Check sheet for the modelled part. Datum: model origin and axes. Units: mm. Face numbers are marked on the shaded views. A direction names the side the tool comes from. Coordinates: 2 decimals unless noted, no trailing zeros. Loops run counter-clockwise (first coordinate to the right, second up) from the corner with the lowest first, then second, coordinate; pieces in that order, holes last. Notation, with made-up numbers: M -38,70 L -6,70 A14 cw -6,92 Z; hole C 32,63 d10. An arc over 180 degrees is marked long. Write each question's results on one line, items separated by ' | '. Start each with the question number.
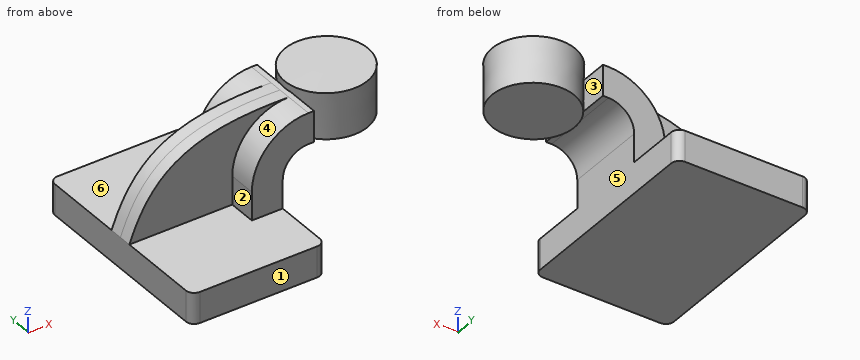
from build123d import *

# Parameters (mm, degrees)
F1_DEPTH = 63.5
F2_DEPTH = 25.4
F3_DEPTH = 7.9375
F5_R     = 5.08


with BuildPart() as f1:
    # F0 (on Front) → F1 (new body, symmetric)
    with BuildSketch(Plane.XZ):
        Polygon((22.2249999642, 9.525), (-41.275, 9.525), (-41.275, -9.525), (41.275, -9.525), (41.275, 9.525), align=None)
    extrude(amount=F1_DEPTH, both=True)

    # F0 (on Front) → F2 (join, symmetric)
    with BuildSketch(Plane.XZ):
        with BuildLine():
            Line((22.2249999642, 27.0002), (22.2249999642, 9.525))
            Line((22.2249999642, 9.525), (41.275, 9.525))
            Line((41.275, 9.525), (41.275, 27.0002))
            ThreePointArc((41.275, 27.0002), (45.9246798487, 38.2255201513), (57.15, 42.8752))
            Line((57.15, 42.8752), (60.587947001, 42.8752))
            Line((60.587947001, 42.8752), (60.587947001, 61.9252000358))
            Line((60.587947001, 61.9252000358), (57.15, 61.9252000358))
            ThreePointArc((57.15, 61.9252000358), (32.4542956418, 51.6959043582), (22.2249999642, 27.0002))
        make_face()
    extrude(amount=F2_DEPTH, both=True)

    # F0 (on Front) → F3 (join, symmetric)
    with BuildSketch(Plane.XZ):
        with BuildLine():
            add(Edge.make_bspline(
                [(-41.275, 9.525), (-27.342395857, 48.1158420444), (-3.4818400163, 63.5879263282), (57.15, 61.9252000358)],
                knots=[0, 0, 0, 0, 111.5045361803, 111.5045361803, 111.5045361803, 111.5045361803], degree=3))
            Line((-41.275, 9.525), (22.2249999642, 9.525))
            Line((22.2249999642, 9.525), (22.2249999642, 27.0002))
            ThreePointArc((22.2249999642, 27.0002), (32.4542956418, 51.6959043582), (57.15, 61.9252000358))
        make_face()
    extrude(amount=F3_DEPTH, both=True)

    # F0 (on Front) → F4 (revolve)
    with BuildSketch(Plane.XZ):
        Polygon((111.387947001, 66.675), (85.725, 66.675), (85.987947001, 38.1), (111.387947001, 38.1), align=None)
    revolve(axis=Axis((85.8564735005, 0, 52.3875), (-0.0092016052, 0, 0.9999576643)))

    # F5
    f5_edges = [f1.edges().sort_by_distance(p)[0] for p in [
        (41.275, -63.5, 0),
        (-41.275, -63.5, 0),
        (41.275, 63.5, 0),
        (-41.275, 63.5, 0),
    ]]
    fillet(f5_edges, radius=F5_R)


solid = f1.part
Item 1: Tool access check on the marked faces 4, 5 and 6. Record the directions out of +Z, -Z, +X, -X, +Y, -Y that give a thin tool (end or side, any length) a straight path to the whole face; none if there is none.
Item 2: Section check B-B (y = -42). Record the cut outline in (x, z) (3 decimals), plus the area to 3 significant figures.
Item 3: Section check A-A (z = 3). Record the cut outline in (x, y) (3 decimals), plus the area to 3 significant figures.
Item 4: Depth check by flat-ended pin: P1, Ø9.5, axis at y = -19.5, z = 54.5, coming from the +X side; P2, Ø4, axis at x = 59.5, y = -4.5, coming from the +Z side; P3, Ø11.5, axis at x = 49, z = 38.5, coming from the -Y side. Enter the tip coordinate at first touch or a pass-through.
Item 5: Thickness scan on line 1 (X direction, y = 27, z = -4.5) (3 decimals); line 2 (Y direction, x = 5.5, z = 11); line 3 (X direction, y = 13, z = 15) (3 decimals). Record the ranges inside material, lowest first.
Item 6: Release check for a two-part mould opening along X. For the marked faces 1, 2 and 3 record: +X half, -X half, draft (parallel to the pull), parting line (faces both ways), or undercut.
Computed values:
1) face 4: +Z, -X, -Y | face 5: -Z, +X, +Y, -Y | face 6: +Z, -X, +Y
2) outline: M -41.275,-9.525 L 41.275,-9.525 L 41.275,9.525 L -41.275,9.525 Z | area: 1,570 mm²
3) outline: M -41.275,-58.42 A5.08 ccw -36.195,-63.5 L 36.195,-63.5 A5.08 ccw 41.275,-58.42 L 41.275,58.42 A5.08 ccw 36.195,63.5 L -36.195,63.5 A5.08 ccw -41.275,58.42 Z | area: 10,500 mm²
4) P1: stops at x = 106.7 | P2: stops at z = 66.23 | P3: stops at y = -25.4
5) line 1: x = -41.275 to 41.275 | line 2: y = -7.94 to 7.94 | line 3: x = 22.225 to 41.275
6) face 1: draft | face 2: -X half | face 3: undercut
